Design review of the part built by this model. Coordinates are the model's own, in mm. A direction names the side the tool comes from. Give positions to 0.01 mm unless a question says otherwise; leave off trailing zeros. Order: outer loops, then holes, each group sorted by start corner. A loop starts at its lowest first (then second) coordinate and runs counter-clockwise, first axis right, second up. Notation, with made-up numbers: (60, 83.5) -> (115, 83.5) arc R29 ccw to (115, 113.5) -> close; hole circle Ø4 at (29, 86). An arc over 180 degrees is marked (long way). Return JSON: item names as keys, results as strings.
```python
from build123d import *

# Parameters (mm, degrees)
BOSS_EXTRUDE1_DEPTH = 120
SKETCH2_W           = 184
SKETCH2_H           = 85
CUT_EXTRUDE1_DEPTH  = 370
SKETCH3_R           = 40.4
CUT_EXTRUDE2_DEPTH  = 8


with BuildPart() as part:
    # Sketch1 → Boss-Extrude1 (new body)
    with BuildSketch(Plane(origin=(0, 0, 0), x_dir=(1, 0, 0), z_dir=(0, 1, 0))):
        with BuildLine():
            Line((0, 120), (-135, 120))
            ThreePointArc((-135, 120), (-138.535533906, 118.535533906), (-140, 115))
            Line((-140, 115), (-140, -115))
            ThreePointArc((-140, -115), (-138.535533906, -118.535533906), (-135, -120))
            Line((-135, -120), (135, -120))
            ThreePointArc((135, -120), (138.535533906, -118.535533906), (140, -115))
            Line((140, -115), (140, 115))
            ThreePointArc((140, 115), (138.535533906, 118.535533906), (135, 120))
            Line((135, 120), (0, 120))
        make_face()
    extrude(amount=BOSS_EXTRUDE1_DEPTH)

    # Sketch2 → Cut-Extrude1 (cut)
    with BuildSketch(Plane(origin=(140, 0, 0), x_dir=(0, 0, -1), z_dir=(1, 0, 0))):
        with Locations((0, 52.5)):
            Rectangle(SKETCH2_W, SKETCH2_H)
    extrude(amount=-CUT_EXTRUDE1_DEPTH, mode=Mode.SUBTRACT)

    # Sketch3 → Cut-Extrude2 (cut)
    with BuildSketch(Plane(origin=(0, 120, 0), x_dir=(1, 0, 0), z_dir=(0, 1, 0))):
        with Locations(Location((70, -45, 0), (0, 0, 270))):
            Circle(SKETCH3_R)
        with Locations(Location((-70, -45, 0), (0, 0, 90))):
            Circle(SKETCH3_R)
        with Locations(Location((0, 60, 0), (0, 0, 270))):
            Circle(SKETCH3_R)
        with Locations(Location((-90.2, 60, 0), (0, 0, 270))):
            Circle(SKETCH3_R)
        with Locations(Location((90.2, 60, 0), (0, 0, 270))):
            Circle(SKETCH3_R)
    extrude(amount=-CUT_EXTRUDE2_DEPTH, mode=Mode.SUBTRACT)


solid = part.part
```
Item 1: For pin 1 (10 mm diameter, centred on y = 64, z = -85, fed in from -X), flat-tipped, find the tip position at first contact; note if it passes through.
Result set:
{"pin 1": "passes through"}
Item 2: Wall thickness on L1, parallel to X at y = 117, z = -60; L2, parallel to X at y = 117.75, z = 45; L3, parallel to Y at x = -34.5, z = -86: over which ranges is each line inside the solid? List them lowest first. Write a range as [from, to].
Result set:
{"L1": "x = [-140, -130.6], [-49.8, -40.4], [40.4, 49.8], [130.6, 140]", "L2": "x = [-140, -110.4], [-29.6, 29.6], [110.4, 140]", "L3": "y = [0, 10], [95, 120]"}
Item 3: Mouldability with a two-part tool opening along Y and no side actions: class faces 4 (the face through (2, 59, -120)), 5 (the face through (2, 52, 92)), 6 (the face through (71, 112, 44)) as released by +Y, released by -Y, zero draft, split by the parting line, or undercut.
Result set:
{"face 4": "zero draft", "face 5": "undercut", "face 6": "released by +Y"}
Item 4: Add section D-D (z = 45). Give the boundary of the cut face in (x, y).
Result set:
{"outline": "(-140, 0) -> (140, 0) -> (140, 10) -> (-140, 10) -> close; (-140, 95) -> (140, 95) -> (140, 120) -> (110.4, 120) -> (110.4, 112) -> (29.6, 112) -> (29.6, 120) -> (-29.6, 120) -> (-29.6, 112) -> (-110.4, 112) -> (-110.4, 120) -> (-140, 120) -> close"}
Item 5: Add section B-B (x = 0). Give the boundary of the cut face in (y, z), plus the area to 3 significant figures.
Result set:
{"outline": "(0, -120) -> (120, -120) -> (120, -100.4) -> (112, -100.4) -> (112, -19.6) -> (120, -19.6) -> (120, 120) -> (0, 120) -> close; hole (10, -92) -> (95, -92) -> (95, 92) -> (10, 92) -> close", "area": "12,500 mm^2"}
Item 6: Add section A-A (z = -60). Give the boundary of the cut face in (x, y).
Result set:
{"outline": "(-140, 0) -> (140, 0) -> (140, 10) -> (-140, 10) -> close; (-140, 95) -> (140, 95) -> (140, 120) -> (130.6, 120) -> (130.6, 112) -> (49.8, 112) -> (49.8, 120) -> (40.4, 120) -> (40.4, 112) -> (-40.4, 112) -> (-40.4, 120) -> (-49.8, 120) -> (-49.8, 112) -> (-130.6, 112) -> (-130.6, 120) -> (-140, 120) -> close"}
Item 7: Add section C-C (y = 84.5). Give the boundary of the cut face in (x, z).
Result set:
{"outline": "(-140, -115) arc R5 ccw to (-135, -120) -> (135, -120) arc R5 ccw to (140, -115) -> (140, -92) -> (-140, -92) -> close; (-140, 92) -> (140, 92) -> (140, 115) arc R5 ccw to (135, 120) -> (-135, 120) arc R5 ccw to (-140, 115) -> close"}
Item 8: Machinability: for faces 1 (the face through (1, 112, -61)), 2 (the face through (-140, 99, -2)), 3 (the face through (2, 52, -92)), which of the approach directions +Z, -Z, +X, -X, +Y, -Y give a long, thin tool a straight path to every point of the face, cutting with its end or side? Answer none if there is none.
Result set:
{"face 1": "+Y", "face 2": "+Z, -Z, -X, +Y, -Y", "face 3": "+X, -X"}
